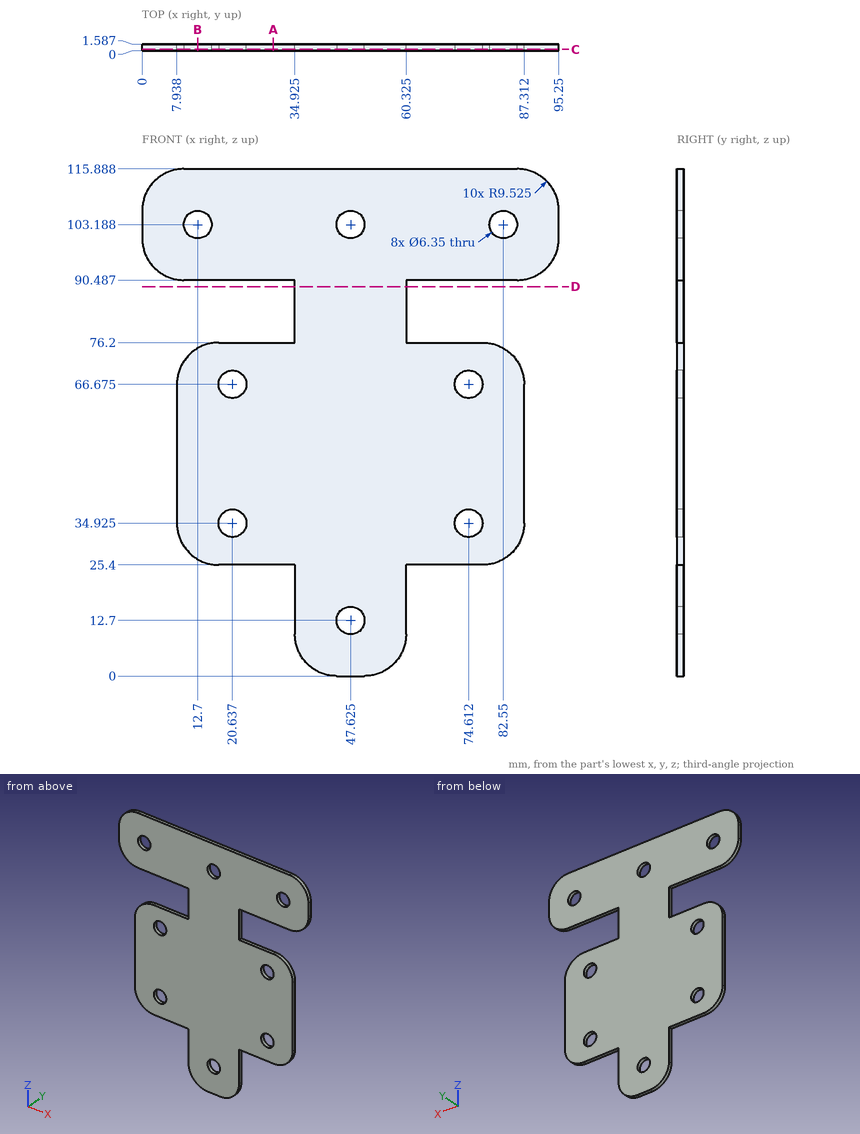
Design review of the part shown in the three views and the two pictorial views. Dimensions are in mm from the part's minimum x, y and z. Round coordinates to 2 decimals unless told otherwise and drop trailing zeros. Write each loop counter-clockwise with the first axis right and the second up, starting at its lowest first coordinate (ties: lowest second). Pieces come first, ordered by that corner, then holes. Notation, with made-up numbers: (81.25, 6) - (126.25, 6) arc R29 cw to (126.25, 39) - close; hole circle Ø1 at (-25.5, 20.5). An arc over 180 degrees is marked (long way). Write item = value, one per line. Start each with the question number.
1. Consider section B-B on x = 12.7. State the section outline as (y, z) points.
2. Consider section D-D on z = 89. State the section outline as (x, y) points (1 decimal).
3. Consider section A-A on x = 30. State the section outline as (y, z) points.
4. For pin 1 Ø0.5 at (x, y) = (71.5, 1) entering from -Z; pin 2 Ø0.5 at (y, z) = (0.5, 84) entering from -X (1 decimal), all flat-tipped, find the tip position at first contact; note any pin that passes through.
5. Consider section C-C on y = 0.35. Give the number of separate pieces and of enclosed holes in the cut face, plus the area to 3 significant figures.
6. Wall thickness on L1, parallel to Z at x = 70, y = 1.5; L2, parallel to Z at x = 14.5, y = 1.35 (1 decimal); L3, parallel to Z at x = 72, y = 1.5 (1 decimal): over which ranges is each line inside the solid? List them lowest first.
Evaluation:
q1.outline = (0, 26.68) - (1.59, 26.68) - (1.59, 74.92) - (0, 74.92) - close; (0, 90.49) - (1.59, 90.49) - (1.59, 100.01) - (0, 100.01) - close; (0, 106.36) - (1.59, 106.36) - (1.59, 115.89) - (0, 115.89) - close
q2.outline = (34.9, 0) - (60.3, 0) - (60.3, 1.6) - (34.9, 1.6) - close
q3.outline = (0, 25.4) - (1.59, 25.4) - (1.59, 76.2) - (0, 76.2) - close; (0, 90.49) - (1.59, 90.49) - (1.59, 115.89) - (0, 115.89) - close
q4.pin_1 = 25.4
q4.pin_2 = 34.9
q5.separate_pieces = 1
q5.enclosed_holes = 8
q5.area = 7,010 mm2
q6.L1 = 25.4 to 76.2, 90.49 to 115.89
q6.L2 = 25.9 to 75.7, 90.5 to 100.6, 105.8 to 115.9
q6.L3 = 25.4 to 33.1, 36.7 to 64.9, 68.5 to 76.2, 90.5 to 115.9
